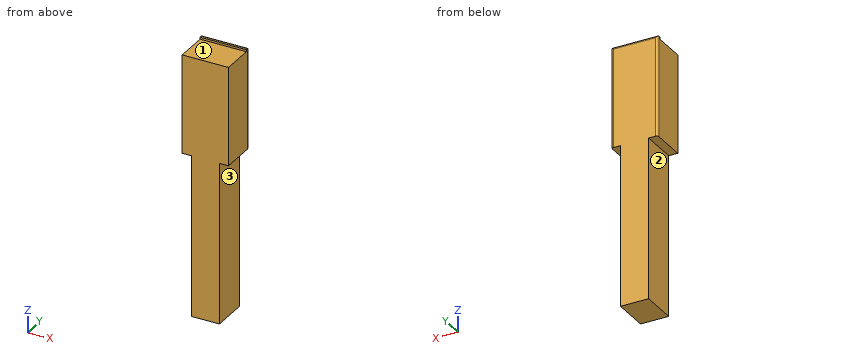
```python
from build123d import *

# Parameters (mm, degrees)
SALIENTE_EXTRUIR1_DEPTH = 18
CROQUIS3_W              = 23
CROQUIS3_H              = 16
CORTAR_EXTRUIR1_DEPTH   = 1
REDONDEO1_R             = 1


with BuildPart() as part:
    # Croquis2 → Saliente-Extruir1 (new body)
    with BuildSketch(Plane(origin=(0, 0, 0), x_dir=(1, 0, 0), z_dir=(0, 1, 0))):
        Polygon((0, 50), (0, 0), (23, 0), (23, 50), (18.5, 50), (18.5, 130), (4.5, 130), (4.5, 50), align=None)
    extrude(amount=SALIENTE_EXTRUIR1_DEPTH)

    # Croquis3 → Cortar-Extruir1 (cut)
    with BuildSketch(Plane.XY):
        with Locations((11.5, 8)):
            Rectangle(CROQUIS3_W, CROQUIS3_H)
    extrude(amount=-CORTAR_EXTRUIR1_DEPTH, mode=Mode.SUBTRACT)

    # Redondeo1
    redondeo1_edges = [part.edges().sort_by_distance(p)[0] for p in [
        (0, 18, -25),
        (11.5, 18, 0),
        (23, 18, -25),
    ]]
    fillet(redondeo1_edges, radius=REDONDEO1_R)


solid = part.part
```
The model under review builds one solid part; all positions refer to its coordinate system, in mm. Face numbers are marked on the shaded views. A direction names the side the tool comes from. Round coordinates to 2 decimals unless told otherwise and drop trailing zeros. Order: outer loops, then holes, each group sorted by start corner. A loop starts at its lowest first (then second) coordinate and runs counter-clockwise, first axis right, second up.
Item 1: To check wall thickness, follow probe 1 along Z at (x, y) = (4, 13.5); probe 2 along Z at (x, y) = (10.75, 7.5); probe 3 along X at (y, z) = (14.25, -90). State the ranges of each line that lie inside material, in increasing order.
Working result:
probe 1: z = -50 to -1
probe 2: z = -130 to -1
probe 3: x = 4.5 to 18.5
Item 2: Add section B-B, the plane z = -109.5. State the section outline as (x, y) points, and give its area (3 significant figures).
Working result:
outline: (4.5, 0) - (18.5, 0) - (18.5, 18) - (4.5, 18) - close
area: 252 mm2
Item 3: Machinability: for the marked faces 1, 2 and 3, which of the approach directions +Z, -Z, +X, -X, +Y, -Y give a long, thin tool a straight path to every point of the face, cutting with its end or side? Answer none if there is none.
Working result:
face 1: +Z, +X, -X, -Y
face 2: -Z, -X, +Y, -Y
face 3: -Z, +X, +Y, -Y
Item 4: For pin 1 (2 mm diameter, centred on y = 4.5, z = -68.5, fed in from -X); pin 2 (0.5 mm diameter, centred on x = 15, z = -0.5, fed in from -Y); pin 3 (1.3 mm diameter, centred on x = 2.5, y = 5.5, fed in from -Z), all flat-tipped, find the tip position at first contact; note any pin that passes through.
Working result:
pin 1: stops at x = 4.5
pin 2: stops at y = 16
pin 3: stops at z = -50
Item 5: Add section A-A, the plane y = 4.5. State the section outline as (x, z) points, and give its area (3 significant figures).
Working result:
outline: (0, -50) - (4.5, -50) - (4.5, -130) - (18.5, -130) - (18.5, -50) - (23, -50) - (23, -1) - (0, -1) - close
area: 2,250 mm2
